```python
from build123d import *

# Parameters (mm, degrees)
EXTRUDE_1_DEPTH     = 20
SKETCH_2_R          = 21
EXTRUDE_2_DEPTH     = 49
SKETCH_3_R          = 12.5
EXTRUDE_3_DEPTH     = 2
SKETCH_4_R          = 4
EXTRUDE_4_DEPTH     = 18.5
SKETCH_5_R          = 1.75
CUT_EXTRUDE_1_DEPTH = 22.5
SKETCH_6_W          = 5
SKETCH_6_H          = 5
CUT_EXTRUDE_2_DEPTH = 8
CHAMFER_1_SIZE      = 1
SKETCH_7_R          = 12
CUT_EXTRUDE_3_DEPTH = 23
EXTRUDE_5_DEPTH     = 20
EXTRUDE_START       = -13
SKETCH_9_R          = 1.75
SKETCH_9_R_2        = 12
EXTRUDE_6_DEPTH     = 13
CUT_EXTRUDE_START   = -18
SKETCH_10_R         = 1.75
CUT_EXTRUDE_4_DEPTH = 18


with BuildPart() as part:
    # 草图1 → 凸台-拉伸1 (new body)
    with BuildSketch(Plane(origin=(0, 0, 0), x_dir=(1, 0, 0), z_dir=(0, 1, 0))):
        with BuildLine():
            Line((16.56992758, 21), (-16.56992758, 21))
            ThreePointArc((-16.56992758, 21), (-18.915106397, 18.915106397), (-21, 16.56992758))
            Line((-21, 16.56992758), (-21, -16.56992758))
            ThreePointArc((-21, -16.56992758), (-18.915106397, -18.915106397), (-16.56992758, -21))
            Line((-16.56992758, -21), (16.56992758, -21))
            ThreePointArc((16.56992758, -21), (18.915106397, -18.915106397), (21, -16.56992758))
            Line((21, -16.56992758), (21, 16.56992758))
            ThreePointArc((21, 16.56992758), (18.915106397, 18.915106397), (16.56992758, 21))
        make_face()
    extrude(amount=EXTRUDE_1_DEPTH)

    # 草图2 → 凸台-拉伸2 (add)
    with BuildSketch(Plane(origin=(0, 20, 0), x_dir=(1, 0, 0), z_dir=(0, 1, 0))):
        with Locations(Location((0, 0, 0), (0, 0, 270))):
            Circle(SKETCH_2_R)
    extrude(amount=EXTRUDE_2_DEPTH)

    # 草图3 → 凸台-拉伸3 (add)
    with BuildSketch(Plane(origin=(0, 69, 0), x_dir=(1, 0, 0), z_dir=(0, 1, 0))):
        with Locations(Location((0, 0, 0), (0, 0, 270))):
            Circle(SKETCH_3_R)
    extrude(amount=EXTRUDE_3_DEPTH)

    # 草图4 → 凸台-拉伸4 (add)
    with BuildSketch(Plane(origin=(0, 71, 0), x_dir=(1, 0, 0), z_dir=(0, 1, 0))):
        with Locations(Location((0, 0, 0), (0, 0, 270))):
            Circle(SKETCH_4_R)
    extrude(amount=EXTRUDE_4_DEPTH)

    # 草图5 → 切除-拉伸1 (cut)
    with BuildSketch(Plane.XZ):
        with Locations(Location((15.5, 15.5, 0), (0, 0, 270))):
            Circle(SKETCH_5_R)
        with Locations(Location((15.5, -15.5, 0), (0, 0, 270))):
            Circle(SKETCH_5_R)
        with Locations(Location((-15.5, -15.5, 0), (0, 0, 270))):
            Circle(SKETCH_5_R)
        with Locations(Location((-15.5, 15.5, 0), (0, 0, 270))):
            Circle(SKETCH_5_R)
    extrude(amount=-CUT_EXTRUDE_1_DEPTH, mode=Mode.SUBTRACT)

    # 草图6 → 切除-拉伸2 (cut)
    with BuildSketch(Plane(origin=(0, 20, 0), x_dir=(1, 0, 0), z_dir=(0, 1, 0))):
        with Locations((-15.5, -15.5)):
            Rectangle(SKETCH_6_W, SKETCH_6_H)
        with Locations((15.5, -15.5)):
            Rectangle(SKETCH_6_W, SKETCH_6_H)
        with Locations((-15.5, 15.5)):
            Rectangle(SKETCH_6_W, SKETCH_6_H)
        with Locations((15.5, 15.5)):
            Rectangle(SKETCH_6_W, SKETCH_6_H)
    extrude(amount=CUT_EXTRUDE_2_DEPTH, mode=Mode.SUBTRACT)

    # 倒角1
    chamfer_1_edges = [part.edges().sort_by_distance(p)[0] for p in [
        (13, 24, -13),
        (-13, 24, -13),
        (-13, 24, 13),
        (13, 24, 13),
    ]]
    chamfer(chamfer_1_edges, length=CHAMFER_1_SIZE)

    # 草图7 → 切除-拉伸3 (cut)
    with BuildSketch(Plane.XZ):
        with Locations(Location((0, 0, 0), (0, 0, 270))):
            Circle(SKETCH_7_R)
    extrude(amount=-CUT_EXTRUDE_3_DEPTH, mode=Mode.SUBTRACT)

    # 草图8 → 凸台-拉伸5 (add)
    with BuildSketch(Plane.XZ.offset(-23)):
        with BuildLine():
            ThreePointArc((2.1, 0), (-1.29614814, -1.652271164), (-0.5, 2.039607805))
            Line((-0.5, 2.039607805), (-0.5, 10.988630488))
            ThreePointArc((-0.5, 10.988630488), (-7.599342077, -7.95298686), (11, 0))
            ThreePointArc((11, 0), (7.95298686, 7.599342077), (0.5, 10.988630488))
            Line((0.5, 10.988630488), (0.5, 2.039607805))
            ThreePointArc((0.5, 2.039607805), (1.652271164, 1.29614814), (2.1, 0))
        make_face()
    extrude(amount=EXTRUDE_5_DEPTH)

    # 草图9 → 凸台-拉伸6 (add)
    with BuildSketch(Plane(origin=(0, 69, 0), x_dir=(1, 0, 0), z_dir=(0, 1, 0)).offset(EXTRUDE_START)):
        with BuildLine():
            Line((-16.56992758, -21), (16.56992758, -21))
            ThreePointArc((16.56992758, -21), (18.915106397, -18.915106397), (21, -16.56992758))
            Line((21, -16.56992758), (21, 16.56992758))
            ThreePointArc((21, 16.56992758), (18.915106397, 18.915106397), (16.56992758, 21))
            Line((16.56992758, 21), (-16.56992758, 21))
            ThreePointArc((-16.56992758, 21), (-18.915106397, 18.915106397), (-21, 16.56992758))
            Line((-21, 16.56992758), (-21, -16.56992758))
            ThreePointArc((-21, -16.56992758), (-18.915106397, -18.915106397), (-16.56992758, -21))
        make_face()
        with Locations(Location((15.5, 15.5, 0), (0, 0, 90))):
            Circle(SKETCH_9_R, mode=Mode.SUBTRACT)
        with Locations(Location((15.5, -15.5, 0), (0, 0, 90))):
            Circle(SKETCH_9_R, mode=Mode.SUBTRACT)
        with Locations(Location((-15.5, 15.5, 0), (0, 0, 90))):
            Circle(SKETCH_9_R, mode=Mode.SUBTRACT)
        with Locations(Location((-15.5, -15.5, 0), (0, 0, 90))):
            Circle(SKETCH_9_R, mode=Mode.SUBTRACT)
        with Locations(Location((0, 0, 0), (0, 0, 90))):
            Circle(SKETCH_9_R_2, mode=Mode.SUBTRACT)
    extrude(amount=EXTRUDE_6_DEPTH)

    # 草图10 → 切除-拉伸4 (cut)
    with BuildSketch(Plane(origin=(0, 69, 0), x_dir=(1, 0, 0), z_dir=(0, 1, 0)).offset(CUT_EXTRUDE_START)):
        with Locations(Location((15.5, -15.5, 0), (0, 0, 90))):
            Circle(SKETCH_10_R)
        with Locations(Location((-15.5, -15.5, 0), (0, 0, 90))):
            Circle(SKETCH_10_R)
        with Locations(Location((-15.5, 15.5, 0), (0, 0, 90))):
            Circle(SKETCH_10_R)
        with Locations(Location((15.5, 15.5, 0), (0, 0, 90))):
            Circle(SKETCH_10_R)
    extrude(amount=CUT_EXTRUDE_4_DEPTH, mode=Mode.SUBTRACT)


solid = part.part
```
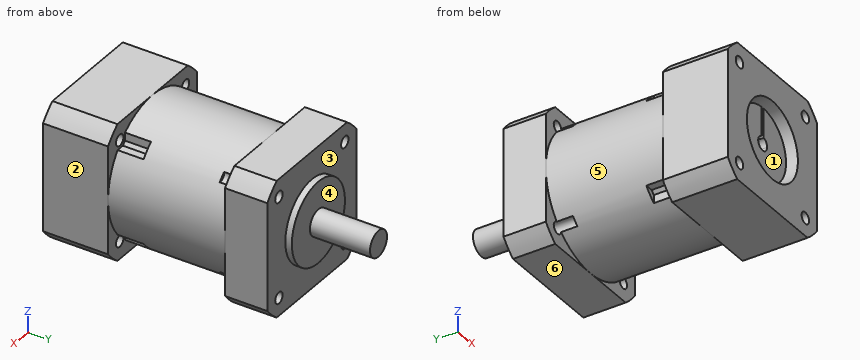
Geometry: final body of the model. Coordinates: model frame, mm. Face numbers are marked on the shaded views. A direction names the side the tool comes from. Coordinates: 2 decimals unless noted, no trailing zeros. Loops run counter-clockwise (first coordinate to the right, second up) from the corner with the lowest first, then second, coordinate; pieces in that order, holes last. Notation, with made-up numbers: (-30, 83.5) -> (-21, 83.5) arc R25 cw to (-21, 101.5) -> close; hole circle Ø4 at (-36.75, -0.75). An arc over 180 degrees is marked (long way). Use a Markdown table: item, result. Add a question column.
(1) Section query C-C, the plane x = -10. Return loops of the section in (y, z).
(2) Mould query, pull axis X, two halves, no side actions, for the marked faces 1, 2 and 3. Classes: pulls with the +X half, pulls with the -X half, needs draft (parallel to the pull), parting line crosses it, or undercut.
(3) Section query A-A, the plane y = 13. Return loops of the section in (x, z), plus the area to 3 significant figures.
(4) Pin query (flat end, axial travel): pin 1 Ø3 at (x, z) = (-15.5, -15.5) entering from -Y; pin 2 Ø4 at (y, z) = (37, -9.5) entering from -X; pin 3 Ø1.2 at (y, z) = (23.5, 15.5) entering from -X. Return the tip coordinate at first contact, or that it passes through.
(5) Section query D-D, the plane y = 59. Return loops of the section in (x, z), plus the area to 3 significant figures.
(6) Line query: line 1 along X through (y, z) = (63, -15.5); line 2 along X through (y, z) = (17, 0); line 3 along Y through (x, z) = (-17.5, -11). Output: solid intervals per line, ascending.
(7) Section query B-B, the plane z = -7. Return loops of the section in (x, y).
(8) Access query for the marked faces 4, 5 and 6. Directions: +Z, -Z, +X, -X, +Y, -Y. A direction counts if a zero-diameter tool reaches every point of the face in a straight line with its end or side. Return the directions, or none.
Answer:
| question | item | result |
|---|---|---|
| 1 | outline | (0, -21) -> (20, -21) -> (20, -18.47) -> (56, -18.47) -> (56, -21) -> (69, -21) -> (69, -7.5) -> (71, -7.5) -> (71, 7.5) -> (69, 7.5) -> (69, 21) -> (56, 21) -> (56, 18.47) -> (20, 18.47) -> (20, 21) -> (0, 21) -> (0, 6.63) -> (23, 6.63) -> (23, 4.58) -> (3, 4.58) -> (3, -4.58) -> (23, -4.58) -> (23, -6.63) -> (0, -6.63) -> close |
| 2 | face 1 | undercut |
| 2 | face 2 | pulls with the +X half |
| 2 | face 3 | needs draft |
| 3 | outline | (-21, -16.57) arc R26.75 ccw to (-16.57, -21) -> (16.57, -21) arc R26.75 ccw to (21, -16.57) -> (21, 16.57) arc R26.75 ccw to (16.57, 21) -> (-16.57, 21) arc R26.75 ccw to (-21, 16.57) -> close; (-0.5, 2.04) -> (-0.5, 10.99) arc R11 ccw (long way) to (0.5, 10.99) -> (0.5, 2.04) arc R2.1 cw (long way) to start; hole circle Ø3.5 at (-15.5, -15.5); hole circle Ø3.5 at (-15.5, 15.5); hole circle Ø24 at (0, 0); hole circle Ø3.5 at (15.5, -15.5); hole circle Ø3.5 at (15.5, 15.5) |
| 3 | area | 1,590 mm^2 |
| 4 | pin 1 | stops at y = 28 |
| 4 | pin 2 | stops at x = -19.62 |
| 4 | pin 3 | stops at x = -13 |
| 5 | outline | (-21, -16.57) arc R26.75 ccw to (-16.57, -21) -> (16.57, -21) arc R26.75 ccw to (21, -16.57) -> (21, 16.57) arc R26.75 ccw to (16.57, 21) -> (-16.57, 21) arc R26.75 ccw to (-21, 16.57) -> close; hole circle Ø3.5 at (-15.5, -15.5); hole circle Ø3.5 at (-15.5, 15.5); hole circle Ø3.5 at (15.5, -15.5); hole circle Ø3.5 at (15.5, 15.5) |
| 5 | area | 1,690 mm^2 |
| 6 | line 1 | x = -21 to -17.25, -13.75 to 13.75, 17.25 to 21 |
| 6 | line 2 | x = -21 to -12, -11 to -2.1, 2.1 to 11, 12 to 21 |
| 6 | line 3 | y = 0 to 69 |
| 7 | outline | (-21, 0) -> (-9.75, 0) -> (-9.75, 23) -> (-8.49, 23) -> (-8.49, 3) -> (8.49, 3) -> (8.49, 23) -> (9.75, 23) -> (9.75, 0) -> (21, 0) -> (21, 20) -> (19.8, 20) -> (19.8, 56) -> (21, 56) -> (21, 69) -> (10.36, 69) -> (10.36, 71) -> (-10.36, 71) -> (-10.36, 69) -> (-21, 69) -> (-21, 56) -> (-19.8, 56) -> (-19.8, 20) -> (-21, 20) -> close |
| 8 | face 4 | +Y |
| 8 | face 5 | none |
| 8 | face 6 | -Z, +X, -X, +Y, -Y |
